Source: CAD feature listing. Evaluate the final solid. Frame: model axes, mm. A direction names the side the tool comes from. Give positions to 0.01 mm unless a question says otherwise; leave off trailing zeros. Order: outer loops, then holes, each group sorted by start corner. A loop starts at its lowest first (then second) coordinate and runs counter-clockwise, first axis right, second up. Notation, with made-up numbers: M 22,-26.5 L 65,-26.5 A13 ccw 65,-9.5 Z; hole C 3,62.25 d3. An arc over 180 degrees is marked long. Use CSV: the item, a comma, the result in double quotes. Start each with the question number.
1. Reachability of faces 1 (the flat face through (5, 0, 63)), 2 (the flat face through (19.93, -0.053, -65.834)), 3 (the cylindrical face through (49.99, -1.05, 1.03)), 4 (the flat face through (30, 0, 68.761)), 5 (the conical face through (13.008, -5.345, -51.848)) from +Z, -Z, +X, -X, +Y, -Y: full face, straight path, thin tool, end or side. Return the list, or none.
2. Section query B-B, the plane x = 28. State how many separate pieces and enclosed holes the cut face has, plus the area to 3 significant figures.
3. Pin query (flat end, axial travel): P1, Ø5, axis at x = 11.5, y = 19.5, coming from the +Z side; P2, Ø6, axis at y = -48.5, z = -31, coming from the +X side; P3, Ø8, axis at x = 34, z = 26.5, coming from the -Y side; P4, Ø5, axis at y = -1.5, z = -60, coming from the +X side. Return the tip coordinate at first contact, or that it passes through.
4. Section query A-A, the plane y = 0. Return the cut outline in (x, z).
5. Line query: line 1 along Z through (x, y) = (32.5, 5); line 2 along Z through (x, y) = (28, -46.5); line 3 along Z through (x, y) = (20, 6). Output: solid intervals per line, ascending. Write a range as [from, to].
6. Mould query, pull axis Z, two halves, no side actions, for faces 6 (the flat face through (13, 3.8, -62)), 7 (the flat face through (30, 0, 76.411)), 8 (the flat face through (30, 0, -76.411)). Classes: released by +Z, released by -Z, zero draft, split by the parting line, or undercut.
from build123d import *

# Parameters (mm, degrees)
SKETCH2_R                 = 52.5
SKETCH2_R_2               = 50
EXTRUDE_THIN1_DEPTH       = 75
CUT_EXTRUDE1_DEPTH        = 75
BOSS_EXTRUDE3_DEPTH       = 10
BOSS_EXTRUDE4_DEPTH       = 50
CHAMFER1_SIZE             = 10
CHAMFER1_SIZE2            = 5.773502691896273
CUT_EXTRUDE2_REACH        = 116.297
SKETCH9_R                 = 2.500000000000002
BOSS_EXTRUDE5_START       = -7.6
BOSS_EXTRUDE5_DEPTH       = 7.6
CHAMFER2_SIZE             = 2.5
CHAMFER1_OF_MIRROR1_SIZE2 = 5.773502691896273
CHAMFER1_OF_MIRROR1_SIZE  = 10
CHAMFER2_OF_MIRROR1_SIZE  = 2.5
CUT_EXTRUDE4_DEPTH        = 55


with BuildPart() as part:
    # Sketch2 → Extrude-Thin1 (new, symmetric)
    with BuildSketch(Plane(origin=(0, 0, 0), x_dir=(1, 0, 0), z_dir=(0, 1, 0))):
        Circle(SKETCH2_R)
        Circle(SKETCH2_R_2, mode=Mode.SUBTRACT)
    extrude(amount=EXTRUDE_THIN1_DEPTH, both=True)

    # Sketch3 → Cut-Extrude1 (cut, symmetric)
    with BuildSketch(Plane(origin=(0, 0, 0), x_dir=(1, 0, 0), z_dir=(0, 1, 0))):
        Polygon((4.999999999999993, 59.38113102411591), (5.000000000000009, -67.26797399217554), (-132.829326150241, 10.543220597022644), align=None)
    extrude(amount=CUT_EXTRUDE1_DEPTH, both=True, mode=Mode.SUBTRACT)

    # Sketch4 → Boss-Extrude3 (add)
    with BuildSketch(Plane.ZY.offset(-5)):
        Polygon((49.749371855331, 3.799999999999979), (49.749371855331, -3.7999999999999963), (52.261362400917186, -3.800000000000001), (68.76136240091718, -3.800000000000007), (68.76136240091718, 3.799999999999994), (52.261362400917186, 3.799999999999984), align=None)
    boss_extrude3 = extrude(amount=-BOSS_EXTRUDE3_DEPTH)

    # Sketch8 → Boss-Extrude4 (add)
    with BuildSketch(Plane.ZY.offset(-5)):
        Polygon((68.76136240091718, 10.999999999999995), (68.76136240091718, 3.799999999999994), (68.76136240091718, -3.800000000000007), (68.76136240091718, -11.000000000000009), (70.16136240091718, -11.000000000000007), (76.41136240091718, -4.750000000000007), (76.41136240091718, 4.7499999999999964), (70.16136240091718, 10.999999999999993), align=None)
    boss_extrude4 = extrude(amount=-BOSS_EXTRUDE4_DEPTH)

    # Chamfer1
    chamfer1_edges = [part.edges().sort_by_distance(p)[0] for p in [
        (15.000000000000009, -6.22e-15, 68.76136240091718),
    ]]
    chamfer1_side = [part.faces().sort_by_distance(p)[0] for p in [
        (31.48437500000001, -7.01e-15, 68.76136240091718),
    ]]
    chamfer(chamfer1_edges, length=CHAMFER1_SIZE, length2=CHAMFER1_SIZE2, reference=chamfer1_side[0])

    # Sketch9 → Cut-Extrude2 (cut, up to next)
    with BuildSketch(Plane(origin=(15, 0, -1.86e-15), x_dir=(-1.2e-16, 0, -1), z_dir=(1, 0, -1.2e-16)), mode=Mode.PRIVATE) as cut_extrude2_sk1:
        with Locations((-59.98785970902089, 0)):
            Circle(SKETCH9_R)
    cut_extrude2_tool1 = extrude(cut_extrude2_sk1.sketch, amount=-CUT_EXTRUDE2_REACH, mode=Mode.PRIVATE) & part.part
    cut_extrude2 = cut_extrude2_tool1.solids().sort_by_distance((15, 0, 59.98786))[0]
    add(cut_extrude2, mode=Mode.SUBTRACT)

    # Sketch10 → Boss-Extrude5 (add)
    with BuildSketch(Plane.XZ.offset(3.799999999999893).offset(BOSS_EXTRUDE5_START)):
        with BuildLine():
            Line((24.999999999999964, 46.1654632815485), (15.000000000000007, 56.98785970902091))
            Line((15.000000000000009, 56.98785970902091), (15.00000000000001, 50.311529493745276))
            ThreePointArc((15.000000000000021, 50.311529493745276), (20.10714963039217, 48.49693324057741), (24.99999999999998, 46.165463281548504))
        make_face()
    boss_extrude5 = extrude(amount=BOSS_EXTRUDE5_DEPTH)

    # Chamfer2
    chamfer2_edges = [part.edges().sort_by_distance(p)[0] for p in [
        (15.30653443854551, 3.800000000000107, 50.219119899512584),
        (15.306534438545505, -3.7999999999998963, 50.219119899512584),
    ]]
    chamfer(chamfer2_edges, length=CHAMFER2_SIZE)

    # Mirror1: Boss-Extrude3, Boss-Extrude4, Cut-Extrude2, Boss-Extrude5 across plane
    add(boss_extrude3.mirror(Plane.XY))
    add(boss_extrude4.mirror(Plane.XY))
    add(cut_extrude2.mirror(Plane.XY), mode=Mode.SUBTRACT)
    add(boss_extrude5.mirror(Plane.XY))

    # Chamfer1 of Mirror1
    chamfer1_of_mirror1_edges = [part.edges().sort_by_distance(p)[0] for p in [
        (15.000000000000009, -6.22e-15, -68.76136240091718),
    ]]
    chamfer(chamfer1_of_mirror1_edges, length=CHAMFER1_OF_MIRROR1_SIZE, length2=CHAMFER1_OF_MIRROR1_SIZE2)

    # Chamfer2 of Mirror1
    chamfer2_of_mirror1_edges = [part.edges().sort_by_distance(p)[0] for p in [
        (15.30653443854551, 3.800000000000107, -50.219119899512584),
        (15.306534438545505, -3.7999999999998963, -50.219119899512584),
    ]]
    chamfer(chamfer2_of_mirror1_edges, length=CHAMFER2_OF_MIRROR1_SIZE)

    # Sketch12 → Cut-Extrude4 (cut, symmetric)
    with BuildSketch(Plane.XY):
        with BuildLine():
            Line((5.000000000000006, 15), (5.000000000000006, 75))
            Line((5.000000000000006, 75), (52.50000000000001, 75))
            add(Edge.make_bspline(
                [(5.000000000000006, 15), (5.000000000000009, 32.56722451667293), (5.644874110491452, 59.48712745969903), (26.937651649578847, 74.99999999999999), (52.50000000000001, 75)],
                knots=[0, 0, 0, 0, 0.46185098317111584, 1, 1, 1, 1], degree=3))
        make_face()
    cut_extrude4 = extrude(amount=CUT_EXTRUDE4_DEPTH, both=True, mode=Mode.SUBTRACT)

    # Mirror4: Cut-Extrude4 across plane
    add(cut_extrude4.mirror(Plane.ZX), mode=Mode.SUBTRACT)


solid = part.part
Result set:
1,face 1,"+Z, -Z, -X, +Y, -Y"
1,face 2,"+X, +Y, -Y"
1,face 3,"-X, +Y, -Y"
1,face 4,"+X"
1,face 5,"+X, -Y"
2,separate pieces,"4"
2,enclosed holes,"0"
2,area,"1,110 mm2"
3,P1,"z = 51.72"
3,P2,"x = 44.41"
3,P3,"through"
3,P4,"x = 15"
4,outline,"M 5,-76.41 L 55,-76.41 L 55,-68.76 L 25,-68.76 L 15,-62.99 L 15,-62.49 L 5,-62.49 Z; M 5,-57.49 L 15,-57.49 L 15,-56.99 L 25,-46.17 A52.5 ccw 25,46.17 L 15,56.99 L 15,57.49 L 5,57.49 L 5,49.75 A50 cw 5,-49.75 Z; M 5,62.49 L 15,62.49 L 15,62.99 L 25,68.76 L 55,68.76 L 55,76.41 L 5,76.41 Z"
5,line 1,"[-76.16, -68.76], [-41.23, -38], [38, 41.23], [68.76, 76.16]"
5,line 2,"[-44.41, -41.42], [41.42, 44.41]"
5,line 3,"[-75.16, -68.76], [-48.87, -45.83], [45.83, 48.87], [68.76, 75.16]"
6,face 6,"undercut"
6,face 7,"released by +Z"
6,face 8,"released by -Z"
